Geometry: final body of the model. Coordinates: model frame, mm. Coordinates: 2 decimals unless noted, no trailing zeros. Loops run counter-clockwise (first coordinate to the right, second up) from the corner with the lowest first, then second, coordinate; pieces in that order, holes last. Notation, with made-up numbers: (34.5, 74.25) -> (59.5, 74.25) arc R24 ccw to (59.5, 112.25) -> close; hole circle Ø8 at (-25, -13). An arc over 180 degrees is marked (long way). One line per item, written item: value. Start each with the question number.
Item 1: Section query A-A on z = -50. Return loops of the section in (x, y), then the cut area to 3 significant figures.
Item 2: Contact query for a flat-ended pin moving along its axis: pin 1 Ø7 at (x, z) = (-9.5, -285) entering from -Y. Output: stop coordinate, or through.
Item 3: Ray query, probe 1 along Z at (x, y) = (-10, 2.75); probe 2 along X at (y, z) = (-1.75, -50); probe 3 along Z at (x, y) = (-12, -4.5). Return the intervals inside material, ascending. Write a range as from..to.
Item 4: Section query B-B on x = -9.5. Return loops of the section in (y, z).
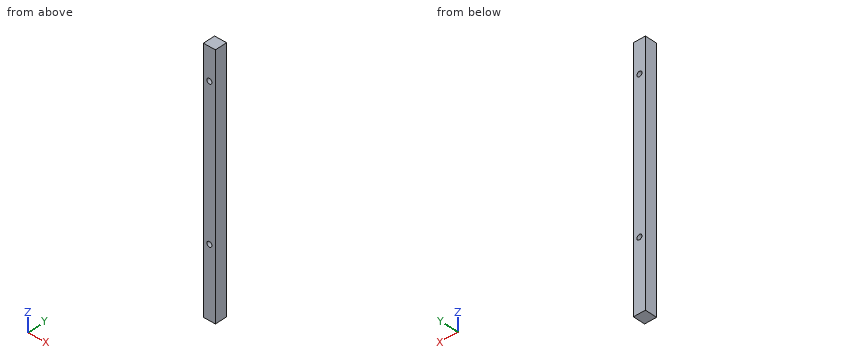
Autodesk Inventor part; units mm, degrees
ref_plane "YZ Plane" through (0, 0, 0) normal (1, 0, 0) x (0, 1, 0)
ref_plane "XZ Plane" through (0, 0, 0) normal (0, 1, 0) x (-1, 0, 0)
ref_plane "XY Plane" through (0, 0, 0) normal (0, 0, 1) x (1, 0, 0)
sketch "Sketch1" plane through (0, 0, 0) normal (0, 1, 0) x (-1, 0, 0)
  line L0 (0, 0) -> (19, 0)
  line L1 (19, 0) -> (19, -395)
  line L2 (19, -395) -> (0, -395)
  line L3 (0, -395) -> (0, 0)
  dimension "d0" = 19
  dimension "d1" = 395
extrude "Extrusion1" add sketch "Sketch1" along normal mid plane 19
sketch "Sketch2" plane through (0, 9.5, 0) normal (0, 1, 0) x (1, 0, 0)
  circle A0 centre (-9.5, 50) radius 4
  circle A1 centre (-9.5, 285) radius 4
  line L0 (-19, 0) -> (0, 0)
  line L1 (-19, 395) -> (-19, 0)
  line L2 (0, 395) -> (-19, 395)
  dimension "d4" = 8
  dimension "d5" = 8
  dimension "d6" = 50
  dimension "d7" = 9.5
  dimension "d8" = 9.5
  dimension "d12" = 235
extrude "Extrusion2" cut sketch "Sketch2" against normal blind 19
properties part number "Base395" material "Steel"
Reply:
1. outline: (-19, -9.5) -> (-13.5, -9.5) -> (-13.5, 9.5) -> (-19, 9.5) -> close; (-5.5, -9.5) -> (0, -9.5) -> (0, 9.5) -> (-5.5, 9.5) -> close
1. area: 209 mm²
2. pin 1: passes through
3. probe 1: z = -395..-288.97, -281.03..-53.97, -46.03..0
3. probe 2: x = -19..-13.5, -5.5..0
3. probe 3: z = -395..-288.12, -281.88..-53.12, -46.88..0
4. outline: (-9.5, -395) -> (9.5, -395) -> (9.5, -289) -> (-9.5, -289) -> close; (-9.5, -281) -> (9.5, -281) -> (9.5, -54) -> (-9.5, -54) -> close; (-9.5, -46) -> (9.5, -46) -> (9.5, 0) -> (-9.5, 0) -> close
